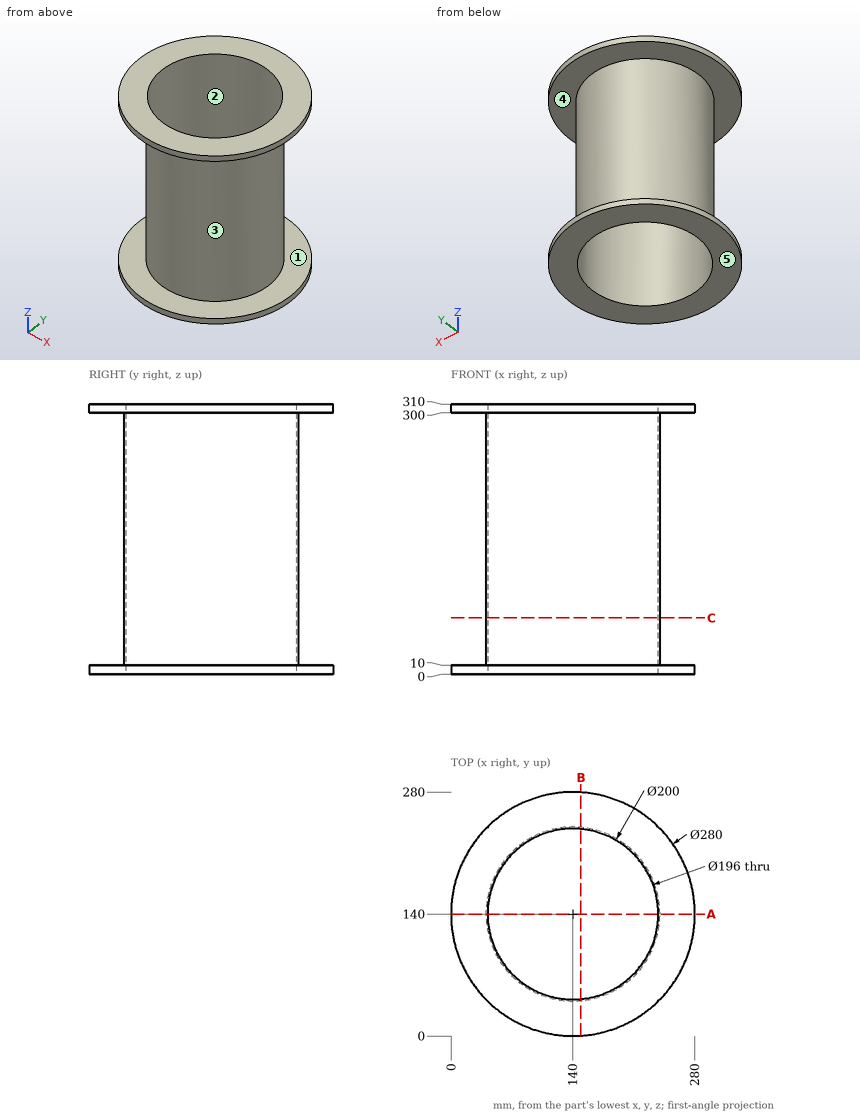
For this review, use the dimensioned drawing (mm, ordinates from the lowest corner) and the shaded views. A direction names the side the tool comes from. Round coordinates to 2 decimals unless told otherwise and drop trailing zeros. Order: outer loops, then holes, each group sorted by start corner. A loop starts at its lowest first (then second) coordinate and runs counter-clockwise, first axis right, second up. Notation, with made-up numbers: (34, 70.25) -> (86, 70.25) arc R23 cw to (86, 93.25) -> close; hole circle Ø4 at (70.5, 74). An arc over 180 degrees is marked (long way). Put each result on its own line as item: value.
Q1. For probe 1 along Y at (x, z) = (140, 88); probe 2 along Z at (x, y) = (38, 53.5); probe 3 along Y at (x, z) = (124, 113.5), list the stretches that pass through material, from the lowest coordinate up. Write a range as [from, to].
Check result:
probe 1: [40, 42], [238, 240]
probe 2: [0, 10], [300, 310]
probe 3: [41.29, 43.31], [236.69, 238.71]
Q2. Add section C-C on z = 64.5. Write out the cut boundary in (x, y), plus the area to 3 significant figures.
Check result:
outline: circle Ø200 at (140, 140); hole circle Ø196 at (140, 140)
area: 1,240 mm2
Q3. Insertion check: pin 1 Ø1.5 at (y, z) = (96, 148) entering from -X; pin 2 Ø10 at (x, z) = (132.5, 200.5) entering from +Y; pin 3 Ø10 at (x, z) = (79.5, 250) entering from +Y; pin 4 Ø10 at (x, y) = (250, 194) entering from -Z. Each pin has a flat end and moves straight along its axis. Give the tip position at first contact, or say it passes through.
Check result:
pin 1: x = 49.84
pin 2: y = 239.97
pin 3: y = 223.19
pin 4: z = 0
Q4. Mouldability with a two-part tool opening along X and no side actions: class the marked faces 1, 2 and 3 as pulls with the +X half, pulls with the -X half, needs draft (parallel to the pull), parting line crosses it, or undercut.
Check result:
face 1: needs draft
face 2: undercut
face 3: parting line crosses it
Q5. Add section B-B on x = 149. Write out the cut boundary in (y, z), plus the area to 3 significant figures.
Check result:
outline: (0.29, 0) -> (42.41, 0) -> (42.41, 310) -> (0.29, 310) -> (0.29, 300) -> (40.41, 300) -> (40.41, 10) -> (0.29, 10) -> close; (237.59, 0) -> (279.71, 0) -> (279.71, 10) -> (239.59, 10) -> (239.59, 300) -> (279.71, 300) -> (279.71, 310) -> (237.59, 310) -> close
area: 2,850 mm2
Q6. Add section A-A on y = 140. Write out the cut boundary in (x, z).
Check result:
outline: (0, 0) -> (42, 0) -> (42, 310) -> (0, 310) -> (0, 300) -> (40, 300) -> (40, 10) -> (0, 10) -> close; (238, 0) -> (280, 0) -> (280, 10) -> (240, 10) -> (240, 300) -> (280, 300) -> (280, 310) -> (238, 310) -> close
Q7. Machinability: for the marked faces 4 and 5, which of the approach directions +Z, -Z, +X, -X, +Y, -Y give a long, thin tool a straight path to every point of the face, cutting with its end or side? Answer none if there is none.
Check result:
face 4: none
face 5: -Z, +X, -X, +Y, -Y
